Build history of the part. All positions in model axes, mm. A direction names the side the tool comes from. Round coordinates to 2 decimals unless told otherwise and drop trailing zeros. Order: outer loops, then holes, each group sorted by start corner. A loop starts at its lowest first (then second) coordinate and runs counter-clockwise, first axis right, second up. Notation, with made-up numbers: M 33,-17 L 69,-17 A19 cw 69,1 Z; hole C 41,1.5 d5. An arc over 180 degrees is marked long. One line per item, written item: value. Start each with the question number.
Item 1: Two-plate mould, pull along Z, no slides. Class faces 4 (the flat face through (111, 12.5, -110)), 5 (the flat face through (108, 3, -24)), 6 (the flat face through (62, 2, 0)): +Z half, -Z half, draft (parallel to the pull), parting line (faces both ways), or undercut.
Item 2: Tool access for faces 1 (the cylindrical face through (106.805, 5.67, -106.259)), 2 (the flat face through (101.263, 3, -61)), 3 (the conical face through (111.95, 12.14, -104.24)): list every direction of +Z, -Z, +X, -X, +Y, -Y with a clear straight run to the whole face (end or side of a thin tool).
Item 3: Band-saw the part on D-D, the plane x = 56. Write the cut outline in (y, z).
Item 4: Band-saw the part on A-A, the plane z = -108.6. Write the cut outline in (x, y).
Item 5: Band-saw the part on B-B, the plane x = 108.6. Write the cut outline in (y, z).
Item 6: Pin check, flat tips, straight feed: pin 1 (5.5 mm diameter, centred on y = 3, z = -15, fed in from -X); pin 2 (3 mm diameter, centred on x = 108.6, z = -108.6, fed in from -Y); pin 3 (5 mm diameter, centred on x = 32, z = -105, fed in from +Y). Stop position of each tip, or through.
Item 7: Probe L1, parallel to X at y = 4, z = -16; L2, parallel to Y at x = 80, z = -10; L3, parallel to Z at x = 65.5, y = 1.75. List the from-to ranges inside material, lowest first.
Item 8: Band-saw the part on C-C, the plane z = -75. Write the cut outline in (x, y).
```python
from build123d import *

# Parameters (mm, degrees)
SKETCH1_W           = 126
SKETCH1_H           = 126
BOSS_EXTRUDE1_DEPTH = 5
SKETCH3_R           = 12.5
BOSS_EXTRUDE2_DEPTH = 7.5
SKETCH4_R           = 2.95
CUT_EXTRUDE1_DEPTH  = 11.5
SKETCH6_R           = 2.5
CUT_EXTRUDE2_DEPTH  = 179.628805068
CHAMFER1_SIZE       = 10
CHAMFER1_SIZE_2     = 7.26542528
SKETCH8_W           = 13
SKETCH8_H           = 63.879672954
SKETCH8_H_2         = 19
CUT_EXTRUDE3_DEPTH  = 179.348675353
SKETCH9_R           = 30
CUT_EXTRUDE4_DEPTH  = 179.348675353


with BuildPart() as part:
    # Sketch1 → Boss-Extrude1 (new body)
    with BuildSketch(Plane(origin=(0, 0, 0), x_dir=(1, 0, 0), z_dir=(0, 1, 0))):
        with Locations((63, 63)):
            Rectangle(SKETCH1_W, SKETCH1_H)
    extrude(amount=BOSS_EXTRUDE1_DEPTH)

    # Sketch3 → Boss-Extrude2 (add)
    with BuildSketch(Plane(origin=(0, 5, 0), x_dir=(1, 0, 0), z_dir=(0, 1, 0))):
        with Locations(Location((108.6, 108.6, 0), (0, 0, 90))):
            Circle(SKETCH3_R)
    extrude(amount=BOSS_EXTRUDE2_DEPTH)

    # Sketch4 → Cut-Extrude1 (cut)
    with BuildSketch(Plane.XZ):
        with Locations(Location((108.6, -108.6, 0), (0, 0, 270))):
            Circle(SKETCH4_R)
    extrude(amount=-CUT_EXTRUDE1_DEPTH, mode=Mode.SUBTRACT)

    # Sketch6 → Cut-Extrude2 (cut, through all)
    with BuildSketch(Plane(origin=(0, 12.5, 0), x_dir=(1, 0, 0), z_dir=(0, 1, 0))):
        with Locations(Location((108.6, 108.6, 0), (0, 0, 270))):
            Circle(SKETCH6_R)
    extrude(amount=-CUT_EXTRUDE2_DEPTH, mode=Mode.SUBTRACT)

    # Chamfer1
    # the kernel refuses this chamfer: 10, 7.26542528 mm, written as the material it takes off along each edge
    with BuildSketch(Plane(origin=(108.6, 12.5, -108.6), x_dir=(0, 0, -1), z_dir=(1, 0, 0))) as chamfer1_piece_1_section:
        Polygon((12.5, -CHAMFER1_SIZE), (12.5 - CHAMFER1_SIZE_2, 0), (12.5, 0), align=None)
    chamfer1_piece_1 = revolve(axis=Axis((108.6, 12.5, -108.6), (0, 1, 0)), mode=Mode.PRIVATE)
    chamfer1_piece_1 = split(chamfer1_piece_1, bisect_by=Plane(origin=(108.6, 5, -100.650989912), z_dir=(0, 1, 0)), keep=Keep.TOP, mode=Mode.PRIVATE)
    add(chamfer1_piece_1, mode=Mode.SUBTRACT)

    # Sketch8 → Cut-Extrude3 (cut, through all)
    with BuildSketch(Plane(origin=(0, 5, 0), x_dir=(1, 0, 0), z_dir=(0, 1, 0))):
        with Locations((107.763328316, 61.0093315)):
            Rectangle(SKETCH8_W, SKETCH8_H)
        with Locations((107.763328316, 14.5)):
            Rectangle(SKETCH8_W, SKETCH8_H_2)
    extrude(amount=-CUT_EXTRUDE3_DEPTH, mode=Mode.SUBTRACT)

    # Sketch9 → Cut-Extrude4 (cut, through all)
    with BuildSketch(Plane(origin=(0, 5, 0), x_dir=(1, 0, 0), z_dir=(0, 1, 0))):
        with Locations(Location((50.837155032, 48.974583989, 0), (0, 0, 270))):
            Circle(SKETCH9_R)
    extrude(amount=-CUT_EXTRUDE4_DEPTH, mode=Mode.SUBTRACT)


solid = part.part
```
Output:
1. face 4: draft
1. face 5: undercut
1. face 6: +Z half
2. face 1: -Y
2. face 2: +Y, -Y
2. face 3: +Y
3. outline: M 0,-126 L 5,-126 L 5,-78.53 L 0,-78.53 Z; M 0,-19.42 L 5,-19.42 L 5,0 L 0,0 Z
4. outline: M 0,0 L 105.65,0 L 105.65,11.5 L 106.1,11.5 L 106.1,12.5 L 103.37,12.5 L 97.92,5 L 0,5 Z; M 111.1,11.5 L 111.55,11.5 L 111.55,0 L 126,0 L 126,5 L 119.28,5 L 113.83,12.5 L 111.1,12.5 Z
5. outline: M 0,-126 L 5,-126 L 5,-119.28 L 12.5,-113.83 L 12.5,-111.1 L 11.5,-111.1 L 11.5,-111.55 L 0,-111.55 Z; M 0,-105.65 L 11.5,-105.65 L 11.5,-106.1 L 12.5,-106.1 L 12.5,-103.37 L 5,-97.92 L 5,-92.95 L 0,-92.95 Z; M 0,-29.07 L 5,-29.07 L 5,-24 L 0,-24 Z; M 0,-5 L 5,-5 L 5,0 L 0,0 Z
6. pin 1: stops at x = 0
6. pin 2: passes through
6. pin 3: stops at y = 5
7. L1: x = 0 to 101.26, 114.26 to 126
7. L2: y = 0 to 5
7. L3: z = -126 to -75.15, -22.8 to 0
8. outline: M 0,0 L 35.91,0 L 35.91,5 L 0,5 Z; M 65.76,0 L 101.26,0 L 101.26,5 L 65.76,5 Z; M 114.26,0 L 126,0 L 126,5 L 114.26,5 Z
